Check sheet for the drawn part. Datum: minimum x, y, z corner. Units: mm. A direction names the side the tool comes from. Coordinates: 2 decimals unless noted, no trailing zeros. Order: outer loops, then holes, each group sorted by start corner. A loop starts at its lowest first (then second) coordinate and runs counter-clockwise, first axis right, second up. Notation, with made-up numbers: M 70.25,21.5 L 105.25,21.5 A16 ccw 105.25,47.5 Z; hole C 51,68.5 d11. An arc over 180 degrees is marked long. Answer in a Markdown table with one row per item. Add a question column.
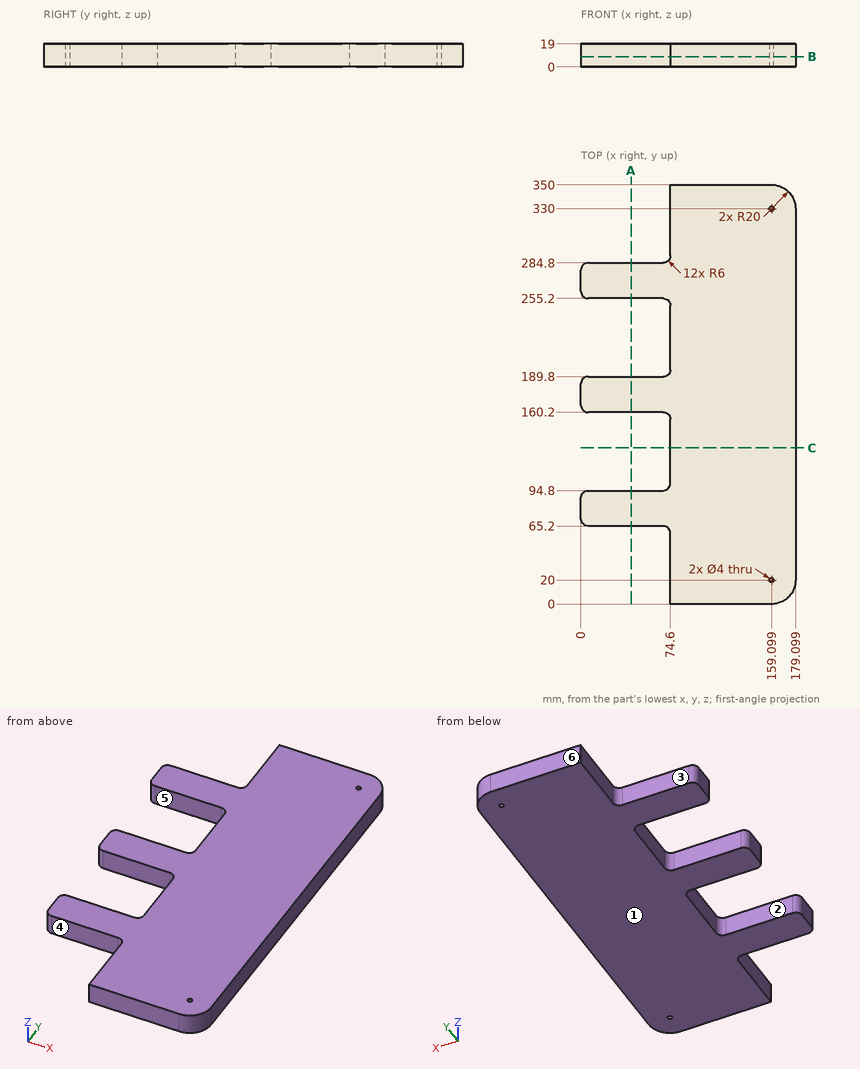
1. Section check B-B on z = 8.5. State how many separate pieces and enclosed holes the cut face has, then the cut area to 3 significant figures.
2. Release check for a two-part mould opening along Y. For the marked faces 4, 5 and 6 record: released by +Y, released by -Y, zero draft, split by the parting line, or undercut.
3. Go/stop test with flat-tipped pins: pin 1 Ø9.5 at (x, z) = (35.5, 13.5) entering from +Y; pin 2 Ø10 at (x, z) = (35.5, 15) entering from -Y; pin 3 Ø5 at (x, z) = (137.5, 7) entering from -Y; pin 4 Ø5.5 at (y, z) = (42.5, 7.5) entering from -X. Record where each tip stops, or that it passes through.
4. Scan lines: line 1 (Y direction, x = 49, z = 9.5); line 2 (X direction, y = 313, z = 18); line 3 (X direction, y = 91, z = 16). Record each from-to range of solid material in increasing order.
5. Section check A-A on x = 42. Enter the section's corners in (y, z).
6. Set-up check for the marked faces 1, 2 and 3: record each of +Z, -Z, +X, -X, +Y, -Y from which the full face is reachable in a straight line by a thin tool's end or side.
7. Section check C-C on y = 130.5. Enter the section's corners in (x, z).
Result sheet:
| question | item | result |
|---|---|---|
| 1 | separate pieces | 1 |
| 1 | enclosed holes | 2 |
| 1 | area | 43,000 mm^2 |
| 2 | face 4 | released by -Y |
| 2 | face 5 | undercut |
| 2 | face 6 | released by +Y |
| 3 | pin 1 | y = 284.8 |
| 3 | pin 2 | y = 65.2 |
| 3 | pin 3 | y = 0 |
| 3 | pin 4 | x = 74.6 |
| 4 | line 1 | 65.2 to 94.8, 160.2 to 189.8, 255.2 to 284.8 |
| 4 | line 2 | 74.6 to 179.1 |
| 4 | line 3 | 0.42 to 179.1 |
| 5 | outline | M 65.2,0 L 94.8,0 L 94.8,19 L 65.2,19 Z; M 160.2,0 L 189.8,0 L 189.8,19 L 160.2,19 Z; M 255.2,0 L 284.8,0 L 284.8,19 L 255.2,19 Z |
| 6 | face 1 | -Z, +X, -X, +Y, -Y |
| 6 | face 2 | +Z, -Z, -X |
| 6 | face 3 | +Z, -Z, -X, +Y |
| 7 | outline | M 74.6,0 L 179.1,0 L 179.1,19 L 74.6,19 Z |
